from build123d import *

# Parameters (mm, degrees)
SKETCH1_R           = 1.6
BOSS_EXTRUDE1_DEPTH = 8.75
FILLET1_R           = 2
CUT_EXTRUDE1_START  = 4.75
CUT_EXTRUDE1_DEPTH  = 3
CUT_EXTRUDE2_START  = -4.75
CUT_EXTRUDE2_DEPTH  = 3
SKETCH3_R           = 2.25
CUT_EXTRUDE3_DEPTH  = 7
SKETCH4_R           = 1.6
BOSS_EXTRUDE3_DEPTH = 0.6


with BuildPart() as part:
    # Sketch1 → Boss-Extrude1 (new, symmetric)
    with BuildSketch(Plane(origin=(0, 0, 0), x_dir=(1, 0, 0), z_dir=(0, 1, 0))):
        with BuildLine():
            Line((0, 5), (-7, 5))
            Line((-7, 5), (-7, -7))
            Line((-7, -7), (5, -7))
            Line((5, -7), (5, 0))
            ThreePointArc((5, 0), (3.535533906, 3.535533906), (0, 5))
        make_face()
        with Locations(Location((0, 0, 0), (0, 0, 270))):
            Circle(SKETCH1_R, mode=Mode.SUBTRACT)
    extrude(amount=BOSS_EXTRUDE1_DEPTH, both=True)

    # Fillet1
    fillet1_edges = [part.edges().sort_by_distance(p)[0] for p in [
        (5, 0, 7),
        (-7, 0, 7),
        (-7, 0, -5),
    ]]
    fillet(fillet1_edges, radius=FILLET1_R)

    # Sketch2 → Cut-Extrude1 (cut)
    with BuildSketch(Plane(origin=(0, 0, 0), x_dir=(1, 0, 0), z_dir=(0, 1, 0)).offset(CUT_EXTRUDE1_START)):
        Polygon((-0.896575472, 3.346065215), (0.757359313, 5), (5, 5), (5, 0.757359313), (3.346065215, -0.896575472), (0.896575472, -3.346065215), (-2.449489743, -2.449489743), (-3.346065215, 0.896575472), align=None)
    extrude(amount=-CUT_EXTRUDE1_DEPTH, mode=Mode.SUBTRACT)

    # Sketch2<2> → Cut-Extrude2 (cut)
    with BuildSketch(Plane(origin=(0, 0, 0), x_dir=(1, 0, 0), z_dir=(0, 1, 0)).offset(CUT_EXTRUDE2_START)):
        Polygon((-0.896575472, 3.346065215), (0.757359313, 5), (5, 5), (5, 0.757359313), (3.346065215, -0.896575472), (0.896575472, -3.346065215), (-2.449489743, -2.449489743), (-3.346065215, 0.896575472), align=None)
    extrude(amount=CUT_EXTRUDE2_DEPTH, mode=Mode.SUBTRACT)

    # Sketch3 → Cut-Extrude3 (cut)
    with BuildSketch(Plane(origin=(0, 8.75, 0), x_dir=(1, 0, 0), z_dir=(0, 1, 0))):
        with Locations(Location((0, 0, 0), (0, 0, 270))):
            Circle(SKETCH3_R)
    extrude(amount=-CUT_EXTRUDE3_DEPTH, mode=Mode.SUBTRACT)

    # Sketch4 → Boss-Extrude3 (add)
    with BuildSketch(Plane.XZ.offset(8.75)):
        with BuildLine():
            Line((10, 0), (10, 5))
            ThreePointArc((10, 5), (7.949747468, 9.949747468), (3, 12))
            Line((3, 12), (-5, 12))
            ThreePointArc((-5, 12), (-9.949747468, 9.949747468), (-12, 5))
            Line((-12, 5), (-12, -3))
            ThreePointArc((-12, -3), (-9.949747468, -7.949747468), (-5, -10))
            Line((-5, -10), (0, -10))
            ThreePointArc((0, -10), (7.071067812, -7.071067812), (10, 0))
        make_face()
        with Locations(Location((0, 0, 0), (0, 0, 270))):
            Circle(SKETCH4_R, mode=Mode.SUBTRACT)
    extrude(amount=-BOSS_EXTRUDE3_DEPTH)


solid = part.part
The model under review builds one solid part; all positions refer to its coordinate system, in mm. A direction names the side the tool comes from. Give positions to 0.01 mm unless a question says otherwise; leave off trailing zeros. Write each loop counter-clockwise with the first axis right and the second up, starting at its lowest first coordinate (ties: lowest second). Pieces come first, ordered by that corner, then holes. Notation, with made-up numbers: M 57,62 L 74,62 A14 cw 74,69 Z; hole C -26.75,79.5 d4. An arc over 180 degrees is marked long. One line per question, with ' | ' between items. Start each with the question number.
Item 1: We need section A-A on y = -1. Write out the cut boundary in (x, z).
Item 2: For pin 1 (4 mm diameter, centred on y = 1, z = 2.5, fed in from +X); pin 2 (1.5 mm diameter, centred on x = 5, y = -1.5, fed in from -Z); pin 3 (9 mm diameter, centred on y = -3.5, z = 2.5, fed in from -X), all flat-tipped, find the tip position at first contact; note any pin that passes through.
Item 3: Draft analysis for pull direction Z (two halves, no side actions). For faces 5 (the cylindrical face through (0.676, 6.778, 2.146)), 6 (the flat face through (5, 0, 3)), 7 (the cylindrical face through (-6.4, 0.42, -4.43)), 8 (the cylindrical face through (8, -8.5, 9.9)), state which applies: released by +Z, released by -Z, zero draft, split by the parting line, or undercut.
Item 4: Wall thickness on line 1 (Y direction, x = 0.25, z = -4.25); line 2 (X direction, y = 6.3, z = 0); line 3 (Y direction, x = -0.75, z = 2): over which ranges is each line inside the solid? List them lowest first. Write a range as from..to.
Item 5: For faces 1 (the flat face through (-0.753, 3.271, 2.904)), 2 (the flat face through (-1.29, 3.27, -2.95)), 3 (the cylindrical face through (4.43, 0.18, 6.4)), 4 (the flat face through (-8, -8.15, 1)), list the 3-axis set-ups (+Z, -Z, +X, -X, +Y, -Y) from which the entire face can be reached by the end or side of a thin tool; tool diameter is ignored.
Item 6: We need section B-B on x = -0.75. Write out the cut boundary in (y, z), plus the area to 3 significant figures.
Item 7: We need section C-C on y = 3. Write out the cut boundary in (x, z), plus the area to 3 significant figures.
Item 8: We need section D-D on y = 6.5. Write out the cut boundary in (x, z), plus the area to 3 significant figures.
Results found:
1) outline: M -7,-3 A2 ccw -5,-5 L 0,-5 A5 ccw 5,0 L 5,5 A2 ccw 3,7 L -5,7 A2 ccw -7,5 Z; hole C 0,0 d3.2
2) pin 1: stops at x = 5 | pin 2: stops at z = -2.63 | pin 3: stops at x = -7
3) face 5: undercut | face 6: zero draft | face 7: released by -Z | face 8: released by +Z
4) line 1: y = -8.75..-4.75, -1.75..1.75, 4.75..8.75 | line 2: x = -7..-2.25, 2.25..5 | line 3: y = -8.75..-4.75, -1.75..1.75
5) face 1: none | face 2: +X | face 3: +Z, +X, +Y | face 4: +Y
6) outline: M -8.75,-10 L -8.15,-10 L -8.15,-5 L 8.75,-5 L 8.75,-2.12 L 4.75,-2.12 L 4.75,-3.49 L 1.75,-3.49 L 1.75,-1.41 L -1.75,-1.41 L -1.75,-3.49 L -4.75,-3.49 L -4.75,-1.41 L -8.75,-1.41 Z; M -8.75,1.41 L -4.75,1.41 L -4.75,2.9 L -1.75,2.9 L -1.75,1.41 L 1.75,1.41 L 1.75,2.9 L 4.75,2.9 L 4.75,2.12 L 8.75,2.12 L 8.75,7 L -8.15,7 L -8.15,12 L -8.75,12 Z | area: 139 mm2
7) outline: M -7,-3 A2 ccw -5,-5 L 0,-5 A5 ccw 0.71,-4.95 L -3.35,-0.9 L -2.45,2.45 L 0.9,3.35 L 4.95,-0.71 A5 ccw 5,0 L 5,5 A2 ccw 3,7 L -5,7 A2 ccw -7,5 Z | area: 92.4 mm2
8) outline: M -7,-3 A2 ccw -5,-5 L 0,-5 A5 ccw 5,0 L 5,5 A2 ccw 3,7 L -5,7 A2 ccw -7,5 Z; hole C 0,0 d4.5 | area: 120 mm2
